The listing builds one solid part. Answer for the finished solid, in the listing's coordinates (mm). A direction names the side the tool comes from. Round coordinates to 2 decimals unless told otherwise and drop trailing zeros. Loops run counter-clockwise (first coordinate to the right, second up) from the corner with the lowest first, then second, coordinate; pieces in that order, holes last. Notation, with made-up numbers: M -9,-36.75 L 5,-36.75 A26 cw 5,-22.75 Z; hole C 34,46.5 d6. An arc over 180 degrees is marked long. Put each result on its own line as item: value. Start each with the question number.
(1) Determine the mould class of faces 1 (the face through (25, 0, 200)), 2 (the face through (895, 25, 507)), 3 (the face through (715, 0, 700)) for opening direction Y: released by +Y, released by -Y, zero draft, split by the parting line, or undercut.
(2) Section A-A, the plane z = 200 is taken. Count the separate pieces of the cut face and the enclosed holes in it, then the cut area to 3 significant figures.
(3) A flat-ended cylindrical pin translates along its axis: P1, Ø13.5, axis at x = 1133, y = -8, coming from the -Z side. Find the tip coordinate at first contact, or state that the pin passes through.
(4) Straight lines are drawn through the part: line 1 (X direction, y = 24.05, z = 40); line 2 (Z direction, x = 1450, y = 24.4); line 3 (X direction, y = -24.2, z = 660). For each, find the intervals that lie inside material, in ascending order.
(5) Section D-D, the plane x = 913.5 is taken. Determine the outline of the cut face in (y, z), then the cut area to 3 significant figures.
(6) Which of the six approach directions +Z, -Z, +X, -X, +Y, -Y give full straight-line access (tool end or side, diameter ignored) to faces 4 (the face through (1450, -23, 355)), 5 (the face through (1230.595, -0.35, 434.525)), 6 (the face through (1448, -24, 0)), 7 (the face through (1290, 0, 223))?
(7) Section B-B, the plane x = 720.5 is taken. Determine the outline of the cut face in (y, z), then the cut area to 3 significant figures.
```python
from build123d import *

# Parameters (mm, degrees)
SKETCH1_W           = 50
SKETCH1_H           = 50
SKETCH1_W_2         = 46
SKETCH1_H_2         = 46
EXTRUDE_THIN1_DEPTH = 700
SKETCH2_W           = 50
SKETCH2_H           = 50
SKETCH2_W_2         = 46
SKETCH2_H_2         = 46
BOSS_EXTRUDE1_DEPTH = 1400
SKETCH4_W           = 50
SKETCH4_H           = 50
SKETCH4_W_2         = 46
SKETCH4_H_2         = 46
EXTRUDE_THIN7_DEPTH = 700
SKETCH6_W           = 50
SKETCH6_H           = 50
SKETCH6_W_2         = 46
SKETCH6_H_2         = 46
BOSS_EXTRUDE2_DEPTH = 1400
SKETCH7_W           = 50
SKETCH7_H           = 50
SKETCH11_W          = 50
SKETCH11_H          = 50
LPATTERN1_COUNT     = 2
LPATTERN1_PITCH     = 747.25
SKETCH17_R          = 17.5
CUT_EXTRUDE1_DEPTH  = 1634.439622392
SKETCH18_R          = 17.5
CUT_EXTRUDE2_DEPTH  = 1634.439622392


with BuildPart() as part:
    # Sketch1 → Extrude-Thin1 (new body)
    with BuildSketch(Plane.XY):
        Rectangle(SKETCH1_W, SKETCH1_H)
        Rectangle(SKETCH1_W_2, SKETCH1_H_2, mode=Mode.SUBTRACT)
    extrude(amount=EXTRUDE_THIN1_DEPTH)

    # Sketch2 → Boss-Extrude1 (add)
    with BuildSketch(Plane(origin=(25, 0, 0), x_dir=(0, 0, -1), z_dir=(1, 0, 0))):
        with Locations((-675, 0)):
            Rectangle(SKETCH2_W, SKETCH2_H)
        with Locations((-675, 0)):
            Rectangle(SKETCH2_W_2, SKETCH2_H_2, mode=Mode.SUBTRACT)
    extrude(amount=BOSS_EXTRUDE1_DEPTH)

    # Sketch4 → Extrude-Thin7 (add)
    with BuildSketch(Plane.XY.offset(700)):
        with Locations((1450, 0)):
            Rectangle(SKETCH4_W, SKETCH4_H)
        with Locations((1450, 0)):
            Rectangle(SKETCH4_W_2, SKETCH4_H_2, mode=Mode.SUBTRACT)
    extrude(amount=-EXTRUDE_THIN7_DEPTH)

    # Sketch6 → Boss-Extrude2 (add)
    with BuildSketch(Plane(origin=(25, 0, 0), x_dir=(0, 0, -1), z_dir=(1, 0, 0))):
        with Locations((-200, 0)):
            Rectangle(SKETCH6_W, SKETCH6_H)
        with Locations((-200, 0)):
            Rectangle(SKETCH6_W_2, SKETCH6_H_2, mode=Mode.SUBTRACT)
    extrude(amount=BOSS_EXTRUDE2_DEPTH)

    # Sweep1: sweep along a path in Sketch10
    with BuildLine(Plane(origin=(753.54174377, 0, -435.057528611), x_dir=(0, 1, 0), z_dir=(-0.8660254037844416, 0, 0.49999999999999495))) as sweep1_path:
        Line((-5.323086145, -1252.91651246), (-5.323086145, -750.433692418))
    # Sketch7 → Sweep1 (sweep)
    with BuildSketch(Plane(origin=(0, 0, 650), x_dir=(-1, 0, 0), z_dir=(0, 0, -1))):
        with Locations((-1380, 0)):
            Rectangle(SKETCH7_W, SKETCH7_H)
    sweep1 = sweep(path=sweep1_path.line)

    # Sweep2: sweep along a path in Sketch12
    with BuildLine(Plane(origin=(895.897459622, 0, 517.246639479), x_dir=(0, -1, 0), z_dir=(-0.8660254037844416, 0, -0.49999999999999495))) as sweep2_path:
        Line((0, -337.457351946), (0, 158.99000514))
    # Sketch11 → Sweep2 (sweep)
    with BuildSketch(Plane.XY.offset(225)):
        with Locations((1064.626135594, 0)):
            Rectangle(SKETCH11_W, SKETCH11_H)
    sweep2 = sweep(path=sweep2_path.line)

    # LPattern1: Sweep1, Sweep2 ×2
    with Locations(*[(-i * LPATTERN1_PITCH, 0, 0) for i in range(1, LPATTERN1_COUNT)]):
        add(sweep1)
        add(sweep2)

    # Sketch17 → Cut-Extrude1 (cut, through all)
    with BuildSketch(Plane.XZ.offset(25)):
        with Locations(Location((0, 660, 0), (0, 0, 270))):
            Circle(SKETCH17_R)
        with Locations(Location((0, 40, 0), (0, 0, 270))):
            Circle(SKETCH17_R)
        with Locations(Location((1450, 40, 0), (0, 0, 270))):
            Circle(SKETCH17_R)
        with Locations(Location((1450, 660, 0), (0, 0, 270))):
            Circle(SKETCH17_R)
    extrude(amount=-CUT_EXTRUDE1_DEPTH, mode=Mode.SUBTRACT)

    # Sketch18 → Cut-Extrude2 (cut, through all)
    with BuildSketch(Plane.XZ.offset(25)):
        with Locations(Location((352.376135594, 200, 0), (0, 0, 270))):
            Circle(SKETCH18_R)
        with Locations(Location((1099.626135594, 200, 0), (0, 0, 270))):
            Circle(SKETCH18_R)
    extrude(amount=-CUT_EXTRUDE2_DEPTH, mode=Mode.SUBTRACT)


solid = part.part
```
Recorded:
1. face 1: undercut
1. face 2: released by +Y
1. face 3: zero draft
2. separate pieces: 4
2. enclosed holes: 2
2. area: 6,090 mm²
3. P1: stops at z = 175
4. line 1: x = -25 to -17.5, 17.5 to 25, 1425 to 1432.5, 1467.5 to 1475
4. line 2: z = 0 to 22.5, 57.5 to 642.5, 677.5 to 700
4. line 3: x = -25 to -17.5, 17.5 to 1432.5, 1467.5 to 1475
5. outline: M -25,175 L 25,175 L 25,225 L -25,225 Z; M -25,443.46 L 25,443.46 L 25,530.06 L -25,530.06 Z; M -25,650 L 25,650 L 25,700 L -25,700 Z; hole M -23,177 L 23,177 L 23,223 L -23,223 Z; hole M -23,652 L 23,652 L 23,698 L -23,698 Z
5. area: 5,100 mm²
6. face 4: +Z, -Z
6. face 5: +Y, -Y
6. face 6: -Z, +X, -X, +Y, -Y
6. face 7: none
7. outline: M -25,175 L 25,175 L 25,225 L -25,225 Z; M -25,650 L 25,650 L 25,700 L -25,700 Z; hole M -23,177 L 23,177 L 23,223 L -23,223 Z; hole M -23,652 L 23,652 L 23,698 L -23,698 Z
7. area: 768 mm²
